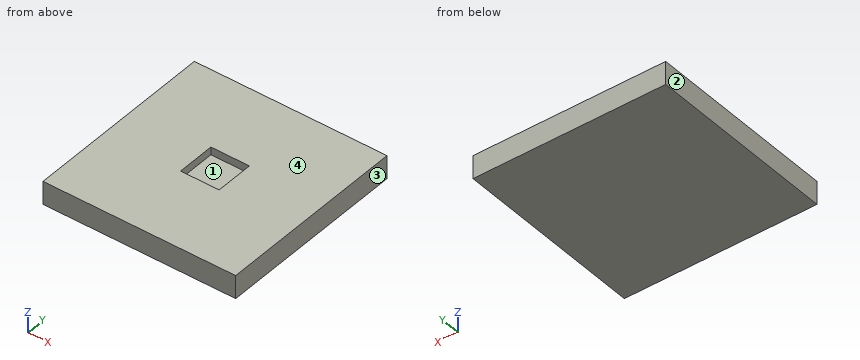
```python
from build123d import *

# Parameters (mm, degrees)
F0_W     = 25
F0_H     = 25
F1_DEPTH = 3
F2_W     = 5
F2_H     = 5
F3_DEPTH = 1


with BuildPart() as f1:
    # F0 (on Top) → F1 (new body)
    with BuildSketch(Plane.XY):
        Rectangle(F0_W, F0_H)
    extrude(amount=F1_DEPTH)


with BuildPart() as f3:
    # F2 (on face) → F3 (new body)
    with BuildSketch(Plane.XY.offset(3)):
        Rectangle(F2_W, F2_H)
    extrude(amount=-F3_DEPTH)


with BuildPart() as f1_1:
    add(f1.part)

    # F4: cut F3
    add(f3.part, mode=Mode.SUBTRACT)


solid = f1_1.part
```
Input: part model. Units: mm. Frame: model coordinates. Face numbers are marked on the shaded views. Coordinates: 2 decimals unless noted, no trailing zeros. Write each loop counter-clockwise with the first axis right and the second up, starting at its lowest first coordinate (ties: lowest second). Pieces come first, ordered by that corner, then holes. Notation, with made-up numbers: (-9.5, -38.5) - (32.5, -38.5) arc R23 cw to (32.5, -8.5) - close; hole circle Ø3 at (85.25, 22.25). An arc over 180 degrees is marked (long way). Put each result on its own line as item: value. Start each with the question number.
1) Contact query for a flat-ended pin moving along its axis: pin 1 (2.5 mm diameter, centred on x = -1, y = 1, fed in from +Z). Output: stop coordinate, or through.
2) Cut plane A-A (x = -0.75). Return the cut outline in (y, z).
3) Ray query, L1, parallel to Y at x = -0.75, z = 2.7. Return the intervals inside material, ascending.
4) Mould query, pull axis X, two halves, no side actions, for the marked faces 1, 2, 3 and 4. Classes: pulls with the +X half, pulls with the -X half, needs draft (parallel to the pull), parting line crosses it, or undercut.
Resolved:
1. pin 1: stops at z = 2
2. outline: (-12.5, 0) - (12.5, 0) - (12.5, 3) - (2.5, 3) - (2.5, 2) - (-2.5, 2) - (-2.5, 3) - (-12.5, 3) - close
3. L1: y = -12.5 to -2.5, 2.5 to 12.5
4. face 1: undercut
4. face 2: pulls with the -X half
4. face 3: pulls with the +X half
4. face 4: needs draft
